from build123d import *

# Parameters (mm, degrees)
F0_W     = 24.087439
F0_H     = 15.245215
F1_DEPTH = 1.5
F2_R     = 0.7
F4_DEPTH = 24.1
F5_R     = 0.7


with BuildPart() as f1:
    # F0 (on Top) → F1 (new body)
    with BuildSketch(Plane.XY):
        with Locations((-20.276139, 22.81383)):
            Rectangle(F0_W, F0_H)
    extrude(amount=F1_DEPTH)

    # F2
    f2_edges = [f1.edges().sort_by_distance(p)[0] for p in [
        (-32.319859, 30.436438, 0.75),
        (-32.319859, 15.191223, 0.75),
        (-8.23242, 30.436438, 0.75),
        (-8.23242, 15.191223, 0.75),
    ]]
    fillet(f2_edges, radius=F2_R)

    # F3 (on face) → F4 (join)
    with BuildSketch(Plane.YZ.offset(-8.23242)):
        Polygon((15.211802, 1.5), (15.891223, 1.5), (30.032871, 6.57918), (29.865546, 7.045054), (15.211802, 1.781947), align=None)
    extrude(amount=-F4_DEPTH)

    # F5
    f5_edges = [f1.edges().sort_by_distance(p)[0] for p in [
        (-32.33242, 29.949209, 6.812117),
        (-8.23242, 29.949209, 6.812117),
    ]]
    fillet(f5_edges, radius=F5_R)


solid = f1.part
Source: CAD feature listing. Evaluate the final solid. Frame: model axes, mm. A direction names the side the tool comes from. Coordinates: 2 decimals unless noted, no trailing zeros. Write each loop counter-clockwise with the first axis right and the second up, starting at its lowest first coordinate (ties: lowest second). Pieces come first, ordered by that corner, then holes. Notation, with made-up numbers: M 25,4 L 48,4 A15 cw 48,17 Z; hole C -30,22.5 d3. An arc over 180 degrees is marked long. Use a Markdown table: item, result.
1) Section B-B, the plane y = 27.5. Output: boundary loops of the cut face in (x, z).
Conclusion:
| item | result |
|---|---|
| outline | M -32.33,5.67 L -8.23,5.67 L -8.23,6.2 L -32.33,6.2 Z; M -32.32,0 L -8.23,0 L -8.23,1.5 L -32.32,1.5 Z |
2) First-contact query: pin 1 Ø1.5 at (x, y) = (-21.5, 26.5) entering from +Z; pin 2 Ø1.5 at (x, y) = (-28, 27.5) entering from +Z; pin 3 Ø4.5 at (x, y) = (-21, 24) entering from +Z. Flat tips, straight axial feed; report the tip coordinate or a pass-through.
Conclusion:
| item | result |
|---|---|
| pin 1 | stops at z = 6.11 |
| pin 2 | stops at z = 6.46 |
| pin 3 | stops at z = 5.75 |
3) Section C-C, the plane z = 5.75. Output: boundary loops of the cut face in (x, y).
Conclusion:
| item | result |
|---|---|
| outline | M -32.33,26.26 L -8.23,26.26 L -8.23,27.72 L -32.33,27.72 Z |
4) Ray query, L1, parallel to Z at x = -17.75, y = 29.5; L2, parallel to Z at x = -9.5, y = 26; L3, parallel to X at y = 19.75, z = 0.5. Return the intervals inside material, ascending.
Conclusion:
| item | result |
|---|---|
| L1 | z = 0 to 1.5, 6.39 to 6.91 |
| L2 | z = 0 to 1.5, 5.13 to 5.66 |
| L3 | x = -32.32 to -8.23 |
5) Reachability of faces 1 (the flat face through (-20, 23, 1.5)), 2 (the flat face through (-20, 23, 0)) from +Z, -Z, +X, -X, +Y, -Y: full face, straight path, thin tool, end or side. Return the list, or none.
Conclusion:
| item | result |
|---|---|
| face 1 | +X, -X, +Y |
| face 2 | -Z, +X, -X, +Y, -Y |
